from build123d import *

# Parameters (mm, degrees)
SKETCH_1_R      = 2
EXTRUDE_1_DEPTH = 300
FILLET_1_R      = 1


with BuildPart() as part:
    # Sketch 1 → Extrude 1 (new body)
    with BuildSketch(Plane.XY):
        Polygon((-20, 10), (-13.9, 10), (-13.9, 8.996845012), (-13.1, 8.996845012), (-13.1, 8), (-16.004631122, 8), (-16.004631122, 6.994580616), (-13.010050506, 4), (-6.989949494, 4), (-3.995368878, 6.994580616), (-3.995368878, 8), (-6.9, 8), (-6.9, 8.996845012), (-6.1, 8.996845012), (-6.1, 10), (6.1, 10), (6.1, 8.996845012), (6.9, 8.996845012), (6.9, 8), (3.995368878, 8), (3.995368878, 6.994580616), (6.989949494, 4), (13.010050506, 4), (16.004631122, 6.994580616), (16.004631122, 8), (13.1, 8), (13.1, 8.996845012), (13.9, 8.996845012), (13.9, 10), (26.1, 10), (26.1, 8.996845012), (26.9, 8.996845012), (26.9, 8), (23.995368878, 8), (23.995368878, 6.994580616), (26.989949494, 4), (33.010050506, 4), (36.004631122, 6.994580616), (36.004631122, 8), (33.1, 8), (33.1, 8.996845012), (33.9, 8.996845012), (33.9, 10), (46.1, 10), (46.1, 8.996845012), (46.9, 8.996845012), (46.9, 8), (43.995368878, 8), (43.995368878, 6.994580616), (46.989949494, 4), (53.010050506, 4), (56.004631122, 6.994580616), (56.004631122, 8), (53.1, 8), (53.1, 8.996845012), (53.9, 8.996845012), (53.9, 10), (60, 10), (60, 3.9), (58.996845012, 3.9), (58.996845012, 3.09747601), (58, 3.09747601), (58, 6), (56.989949494, 6), (54, 3.010050506), (54, -3.010050506), (56.989949494, -6), (58, -6), (58, -3.09747601), (58.996845012, -3.09747601), (58.996845012, -3.9), (60, -3.9), (60, -10), (53.9, -10), (53.9, -8.996845012), (53.1, -8.996845012), (53.1, -8), (56.004631122, -8), (56.004631122, -6.994580616), (53.010050506, -4), (46.989949494, -4), (43.995368878, -6.994580616), (43.995368878, -8), (46.9, -8), (46.9, -8.996845012), (46.1, -8.996845012), (46.1, -10), (33.9, -10), (33.9, -8.996845012), (33.1, -8.996845012), (33.1, -8), (36.004631122, -8), (36.004631122, -6.994580616), (33.010050506, -4), (26.989949494, -4), (23.995368878, -6.994580616), (23.995368878, -8), (26.9, -8), (26.9, -8.996845012), (26.1, -8.996845012), (26.1, -10), (13.9, -10), (13.9, -8.996845012), (13.1, -8.996845012), (13.1, -8), (16.004631122, -8), (16.004631122, -6.994580616), (13.010050506, -4), (6.989949494, -4), (3.995368878, -6.994580616), (3.995368878, -8), (6.9, -8), (6.9, -8.996845012), (6.1, -8.996845012), (6.1, -10), (-6.1, -10), (-6.1, -8.996845012), (-6.9, -8.996845012), (-6.9, -8), (-3.995368878, -8), (-3.995368878, -6.994580616), (-6.989949494, -4), (-13.010050506, -4), (-16.004631122, -6.994580616), (-16.004631122, -8), (-13.1, -8), (-13.1, -8.996845012), (-13.9, -8.996845012), (-13.9, -10), (-20, -10), (-20, -3.9), (-18.996845012, -3.9), (-18.996845012, -3.09747601), (-18, -3.09747601), (-18, -6), (-16.989949494, -6), (-14, -3.010050506), (-14, 3.010050506), (-16.989949494, 6), (-18, 6), (-18, 3.09747601), (-18.996845012, 3.09747601), (-18.996845012, 3.9), (-20, 3.9), align=None)
        with Locations((-10, 0)):
            Circle(SKETCH_1_R, mode=Mode.SUBTRACT)
        with Locations((10, 0)):
            Circle(SKETCH_1_R, mode=Mode.SUBTRACT)
        with Locations((30, 0)):
            Circle(SKETCH_1_R, mode=Mode.SUBTRACT)
        with Locations((50, 0)):
            Circle(SKETCH_1_R, mode=Mode.SUBTRACT)
        Polygon((17.984530109, -6.994580616), (17.984530109, -8), (22.015469891, -8), (22.015469891, -6.994580616), (26, -3.010050506), (26, 3.010050506), (22.015469891, 6.994580616), (22.015469891, 8), (17.984530109, 8), (17.984530109, 6.994580616), (14, 3.010050506), (14, -3.010050506), align=None, mode=Mode.SUBTRACT)
        Polygon((2.015469891, -8), (2.015469891, -6.994580616), (6, -3.010050506), (6, 3.010050506), (2.015469891, 6.994580616), (2.015469891, 8), (-2.015469891, 8), (-2.015469891, 6.994580616), (-6, 3.010050506), (-6, -3.010050506), (-2.015469891, -6.994580616), (-2.015469891, -8), align=None, mode=Mode.SUBTRACT)
        Polygon((42.015469891, -8), (37.984530109, -8), (37.984530109, -6.994580616), (34, -3.010050506), (34, 3.010050506), (37.984530109, 6.994580616), (37.984530109, 8), (42.015469891, 8), (42.015469891, 6.994580616), (46, 3.010050506), (46, -3.010050506), (42.015469891, -6.994580616), align=None, mode=Mode.SUBTRACT)
    extrude(amount=EXTRUDE_1_DEPTH)

    # Fillet 1
    fillet_1_edges = [part.edges().sort_by_distance(p)[0] for p in [
        (60, 10, 150),
        (60, -10, 150),
        (-20, -10, 150),
        (-20, 10, 150),
    ]]
    fillet(fillet_1_edges, radius=FILLET_1_R)


solid = part.part
Model file for the job. Use its own axes, mm. A direction names the side the tool comes from. Coordinates: 2 decimals unless noted, no trailing zeros. Return JSON: item names as keys, results as strings. Group by question number.
Item 1: Flat gauge pins, fed straight in: P1, Ø1.5, axis at x = -11.5, z = 150, coming from the -Y side; P2, Ø1.1, axis at y = -9.5, z = 171, coming from the +X side; P3, Ø0.8, axis at y = -9.5, z = 154.5, coming from the -X side (3 decimals); P4, Ø5, axis at y = 1, z = 137.5, coming from the +X side. Where does each tip first touch, or does it go through?
Item 2: Pull direction X, two halves, no side cores. Call faces 1 (the flat face through (60, 6, 148)), 2 (the flat face through (-20, -6, 148)), 3 (the flat face through (40, -10, 148)), 4 (the flat face through (-10, 4, 148)): pulls with the +X half, pulls with the -X half, needs draft (parallel to the pull), parting line crosses it, or undercut.
Item 3: Wall check: line 1 along X through (y, z) = (2.25, 196); line 2 along Y through (x, z) = (10, 115); line 3 along Y through (x, z) = (25, 146.5). Give the ranges that are in metal, low to high. Write a range as [from, to].
Item 4: Tool access for faces 5 (the flat face through (50, -4, 148)), 6 (the flat face through (14, 0, 148)), 7 (the flat face through (20, 10, 148)), 8 (the flat face through (10, 4, 148)): list every direction of +Z, -Z, +X, -X, +Y, -Y with a clear straight run to the whole face (end or side of a thin tool).
Item 5: Saw through at A-A on z = 52.5. State how many separate pieces and enclosed holes the cut face has, then the cut area to 3 significant figures.
Values found:
{
 "1": {"P1": "stops at y = -4", "P2": "stops at x = 60", "P3": "stops at x = -19.995", "P4": "stops at x = 59"},
 "2": {"face 1": "pulls with the +X half", "face 2": "pulls with the -X half", "face 3": "needs draft", "face 4": "undercut"},
 "3": {"line 1": "x = [-14, -6], [6, 14], [26, 34], [46, 54]", "line 2": "y = [-4, -2], [2, 4]", "line 3": "y = [-10, -8], [-5.99, -4.01], [4.01, 5.99], [8, 10]"},
 "4": {"face 5": "+Z, -Z, -Y", "face 6": "+Z, -Z", "face 7": "+Z, -Z, +X, -X, +Y", "face 8": "+Z, -Z, +Y"},
 "5": {"separate pieces": "1", "enclosed holes": "7", "area": "585 mm2"}
}
